Answer from the drawing. Dimensions are ordinates in mm from the lowest x, y and z of the part. A direction names the side the tool comes from. Give positions to 0.01 mm unless a question says otherwise; leave off trailing zeros. Loops run counter-clockwise (first coordinate to the right, second up) from the corner with the lowest first, then second, coordinate; pieces in that order, holes last.
(1) Determine the mould class of the marked faces 1, 2, 3 and 4 for opening direction X: pulls with the +X half, pulls with the -X half, needs draft (parallel to the pull), parting line crosses it, or undercut.
(2) Find section B-B, the plane y = 47. Write down the section's boundary in (x, z) (1 decimal).
(3) Find section A-A, the plane z = 37. Write down the section's boundary in (x, y) (1 decimal).
(4) Straight lines are drawn through the part: probe 1 along X at (y, z) = (13.5, 31) (1 decimal); probe 2 along Z at (x, y) = (38.5, 39). For each, find the intervals that lie inside material, in ascending order.
(5) Find section C-C, the plane z = 27.5. Write down the section's boundary in (x, y) (1 decimal).
(6) Which of the six approach directions +Z, -Z, +X, -X, +Y, -Y give full straight-line access (tool end or side, diameter ignored) to the marked faces 5 and 6?
(7) Find section D-D, the plane x = 64.5. Write down the section's boundary in (y, z).
(8) This flat-tipped pin is pushed along its axis until it touches: P1, Ø8, axis at x = 61.5, y = 8.5, coming from the -Z side. Where does it stop, or does it pass through?
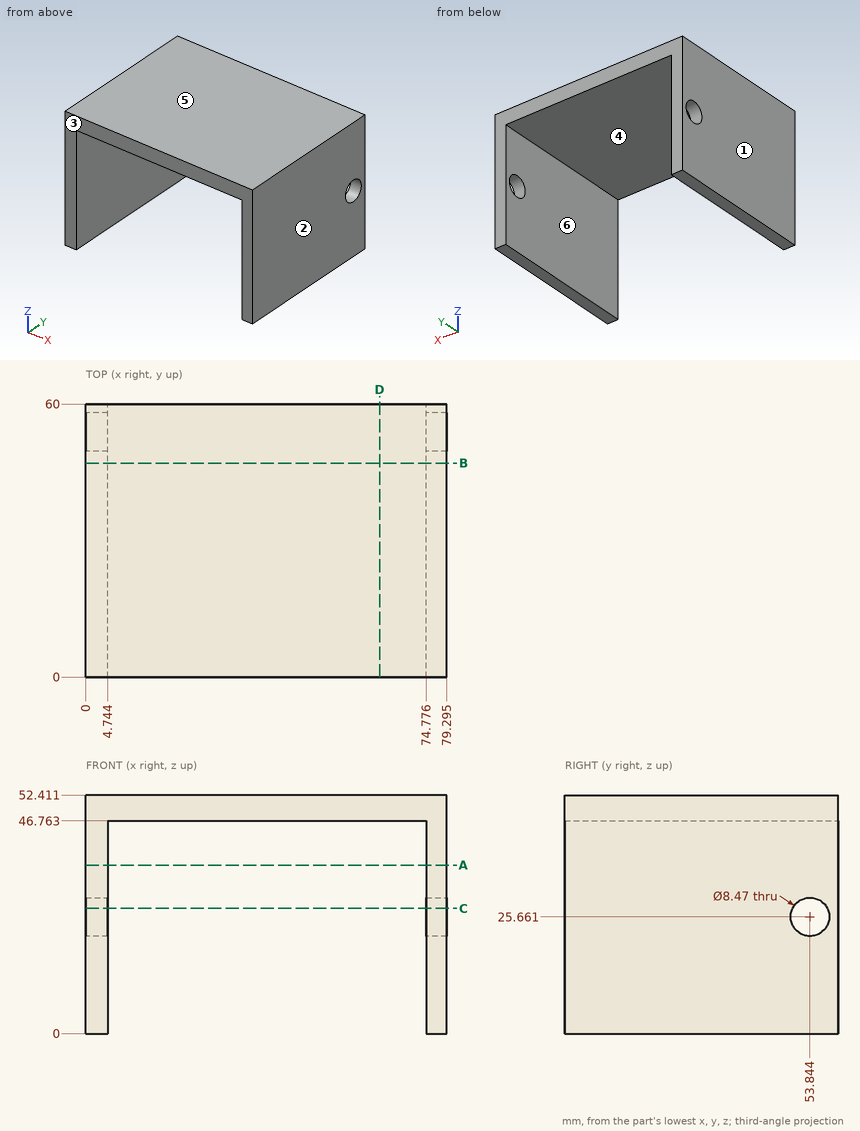
Entries:
1. face 1: pulls with the -X half
1. face 2: pulls with the +X half
1. face 3: needs draft
1. face 4: undercut
2. outline: (0, 0) - (4.7, 0) - (4.7, 46.8) - (74.8, 46.8) - (74.8, 0) - (79.3, 0) - (79.3, 52.4) - (0, 52.4) - close
3. outline: (0, 0) - (4.7, 0) - (4.7, 60) - (0, 60) - close; (74.8, 0) - (79.3, 0) - (79.3, 60) - (74.8, 60) - close
4. probe 1: x = 0 to 4.7, 74.8 to 79.3
4. probe 2: z = 46.76 to 52.41
5. outline: (0, 0) - (4.7, 0) - (4.7, 50) - (0, 50) - close; (0, 57.7) - (4.7, 57.7) - (4.7, 60) - (0, 60) - close; (74.8, 0) - (79.3, 0) - (79.3, 50) - (74.8, 50) - close; (74.8, 57.7) - (79.3, 57.7) - (79.3, 60) - (74.8, 60) - close
6. face 5: +Z, +X, -X, +Y, -Y
6. face 6: -Z, +Y, -Y
7. outline: (0, 46.76) - (60, 46.76) - (60, 52.41) - (0, 52.41) - close
8. P1: stops at z = 46.76
